Part model, mm, in its own coordinate system. Face numbers are marked on the shaded views. A direction names the side the tool comes from. Round coordinates to 2 decimals unless told otherwise and drop trailing zeros. Write each loop counter-clockwise with the first axis right and the second up, starting at its lowest first coordinate (ties: lowest second). Pieces come first, ordered by that corner, then holes. Notation, with made-up numbers: (59, 69) -> (111, 69) arc R29 ccw to (111, 102) -> close; hole circle Ø10 at (19, 79). An arc over 180 degrees is marked (long way). Return JSON: item names as keys, results as strings. Group by question number.
(1) Saw through at B-B (x = 6.25). List the corners of the cut face in (y, z), plus the area to 3 significant figures.
(2) Drop flat-ended pins along their axis: pin 1 Ø1.1 at (x, y) = (7, 4.5) entering from -Z; pin 2 Ø1.6 at (x, y) = (1, 8) entering from +Z; pin 3 Ø1.5 at (y, z) = (7, 2.5) entering from -X. Give the stop position or say it passes through.
(3) Saw through at A-A (y = 5.5). List the corners of the cut face in (x, z).
(4) Tool access for the marked faces 1, 2 and 3: list every direction of +Z, -Z, +X, -X, +Y, -Y with a clear straight run to the whole face (end or side of a thin tool).
(5) Drill centre lines: L1, parallel to Z at x = 1.75, y = 7; L2, parallel to Z at x = 6.75, y = 7; L3, parallel to X at y = 14, z = 1. Where is each one in solid material? Low to high. Write a range as from..to.
(6) Saw through at C-C (z = 0.4). List the corners of the cut face in (x, y), plus the area to 3 significant figures.
from build123d import *

# Parameters (mm, degrees)
SKETCH1_W                    = 4
SKETCH1_H                    = 15
BASE_FLANGE1_DEPTH           = 1
EDGE_FLANGE1_STRIP_W         = 5.4732
EDGE_FLANGE1_STRIP_H         = 1
EDGE_FLANGE1_STRIP_CUT_DEPTH = 15
EDGE_FLANGE1_DEPTH           = 15
EDGE_FLANGE2_STRIP_W         = 5.4732
EDGE_FLANGE2_STRIP_H         = 1
EDGE_FLANGE2_STRIP_CUT_DEPTH = 15
EDGE_FLANGE2_DEPTH           = 15


# Sheet-metal steps are written as plain solids
with BuildPart() as part:
    # Sketch1 → Base-Flange1 (new body)
    with BuildSketch(Plane.XY):
        with Locations((2, 7.5)):
            Rectangle(SKETCH1_W, SKETCH1_H)
    extrude(amount=-BASE_FLANGE1_DEPTH)

    # Edge-Flange1 strip (across the edge) → Edge-Flange1 strip cut (cut)
    with BuildSketch(Plane(origin=(4, 0, 0), x_dir=(-1, 0, 0), z_dir=(0, 1, 0))):
        with Locations((-2, -0.5)):
            Rectangle(EDGE_FLANGE1_STRIP_W, EDGE_FLANGE1_STRIP_H)
    extrude(amount=EDGE_FLANGE1_STRIP_CUT_DEPTH, mode=Mode.SUBTRACT)

    # Edge-Flange1 section (across the edge) → Edge-Flange1 (add)
    with BuildSketch(Plane(origin=(4, 0, 0), x_dir=(-1, 0, 0), z_dir=(0, 1, 0))):
        with BuildLine():
            Line((-1, 0.7366), (-1, 2))
            Line((-1, 2), (0, 2))
            Line((0, 2), (0, 0.7366))
            ThreePointArc((0, 0.7366), (0.215745145, 0.215745145), (0.7366, 0))
            Line((0.7366, 0), (0.7366, -1))
            ThreePointArc((0.7366, -1), (-0.491361636, -0.491361636), (-1, 0.7366))
        make_face()
    extrude(amount=EDGE_FLANGE1_DEPTH)

    # Edge-Flange2 strip (across the edge) → Edge-Flange2 strip cut (cut)
    with BuildSketch(Plane(origin=(5, 15, 2), x_dir=(0, 0, -1), z_dir=(0, -1, 0))):
        with Locations((-2, -0.5)):
            Rectangle(EDGE_FLANGE2_STRIP_W, EDGE_FLANGE2_STRIP_H)
    extrude(amount=EDGE_FLANGE2_STRIP_CUT_DEPTH, mode=Mode.SUBTRACT)

    # Edge-Flange2 section (across the edge) → Edge-Flange2 (add)
    with BuildSketch(Plane(origin=(5, 15, 2), x_dir=(0, 0, -1), z_dir=(0, -1, 0))):
        with BuildLine():
            Line((-1, 0.7366), (-1, 3))
            Line((-1, 3), (0, 3))
            Line((0, 3), (0, 0.7366))
            ThreePointArc((0, 0.7366), (0.215745145, 0.215745145), (0.7366, 0))
            Line((0.7366, 0), (0.7366, -1))
            ThreePointArc((0.7366, -1), (-0.491361636, -0.491361636), (-1, 0.7366))
        make_face()
    extrude(amount=EDGE_FLANGE2_DEPTH)


solid = part.part
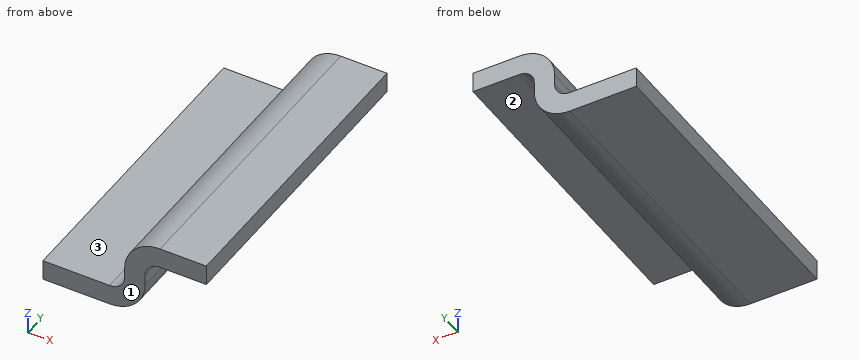
Computed values:
{
 "1": {"outline": "(0, 2) -> (15, 2) -> (15, 3) -> (0, 3) -> close", "area": "15.0 mm2"},
 "2": {"pin 1": "z = 2", "pin 2": "z = 0", "pin 3": "x = 4.07"},
 "3": {"outline": "(0, -1) -> (3.26, -1) arc R1.74 ccw to (5, 0.74) -> (5, 1.26) arc R0.74 cw to (5.74, 2) -> (8, 2) -> (8, 3) -> (5.74, 3) arc R1.74 ccw to (4, 1.26) -> (4, 0.74) arc R0.74 cw to (3.26, 0) -> (0, 0) -> close"},
 "4": {"face 1": "+Z, -Z, +X, -X, -Y", "face 2": "-Z, +X, +Y, -Y", "face 3": "+Z, -X, +Y, -Y"},
 "5": {"L1": "-1..0", "L2": "2..3", "L3": "4..5"},
 "6": {"outline": "(3.92, 0) -> (4.97, 0) -> (4.97, 15) -> (3.92, 15) -> close", "area": "15.7 mm2"}
}
